Read the model definition and answer for the solid it produces. Units are mm, in the model's axes. Face numbers are marked on the shaded views. Coordinates: 2 decimals unless noted, no trailing zeros. Loops run counter-clockwise (first coordinate to the right, second up) from the corner with the lowest first, then second, coordinate; pieces in that order, holes last. Notation, with made-up numbers: (-35, -15) - (20, -15) arc R13 ccw to (20, 8) - close; hole circle Ø4 at (-1, 27). An arc over 180 degrees is marked (long way). Use one line per item in the form item = value.
from build123d import *

# Parameters (mm, degrees)
F1_DEPTH = 12.7
F2_DEPTH = 75.692
F4_DEPTH = 12.7


with BuildPart() as f1:
    # F0 (on Top) → F1 (new body)
    with BuildSketch(Plane.XY):
        with BuildLine():
            ThreePointArc((0, 8.0484505981), (5.691113996, 5.691113996), (8.0484505981, 0))
            ThreePointArc((8.0484505981, 0), (5.691113996, -5.691113996), (0, -8.0484505981))
            Line((0, -8.0484505981), (0, -19.3179212511))
            ThreePointArc((0, -19.3179212511), (13.6598331151, -13.6598331151), (19.3179212511, 0))
            ThreePointArc((19.3179212511, 0), (13.6598331151, 13.6598331151), (0, 19.3179212511))
            Line((0, 19.3179212511), (0, 8.0484505981))
        make_face()
        with BuildLine():
            ThreePointArc((0, -8.0484505981), (-8.0484505981, 0), (0, 8.0484505981))
            Line((0, 8.0484505981), (0, 19.3179212511))
            ThreePointArc((0, 19.3179212511), (-19.3179212511, 0), (0, -19.3179212511))
            Line((0, -19.3179212511), (0, -8.0484505981))
        make_face()
        with BuildLine():
            Line((61.3472089171, 19.3179212511), (0, 19.3179212511))
            ThreePointArc((0, 19.3179212511), (13.6598331151, 13.6598331151), (19.3179212511, 0))
            ThreePointArc((19.3179212511, 0), (13.6598331151, -13.6598331151), (0, -19.3179212511))
            Line((0, -19.3179212511), (61.3472089171, -19.3179212511))
            ThreePointArc((61.3472089171, -19.3179212511), (42.0292876661, 0), (61.3472089171, 19.3179212511))
        make_face()
        with BuildLine():
            ThreePointArc((80.6651301682, 0), (75.0070420322, 13.6598331151), (61.3472089171, 19.3179212511))
            Line((61.3472089171, 19.3179212511), (61.3472089171, 8.0518))
            ThreePointArc((61.3472089171, 8.0518), (67.0406912979, 5.6934823808), (69.3990089171, 0))
            ThreePointArc((69.3990089171, 0), (67.0406912979, -5.6934823808), (61.3472089171, -8.0518))
            Line((61.3472089171, -8.0518), (61.3472089171, -19.3179212511))
            ThreePointArc((61.3472089171, -19.3179212511), (75.0070420322, -13.6598331151), (80.6651301682, 0))
        make_face()
        with BuildLine():
            Line((61.3472089171, 8.0518), (61.3472089171, 19.3179212511))
            ThreePointArc((61.3472089171, 19.3179212511), (42.0292876661, 0), (61.3472089171, -19.3179212511))
            Line((61.3472089171, -19.3179212511), (61.3472089171, -8.0518))
            ThreePointArc((61.3472089171, -8.0518), (53.2954089171, 0), (61.3472089171, 8.0518))
        make_face()
    extrude(amount=F1_DEPTH)

    # F0 (on Top) → F2 (join)
    with BuildSketch(Plane.XY):
        with BuildLine():
            ThreePointArc((0, -8.0484505981), (-8.0484505981, 0), (0, 8.0484505981))
            Line((0, 8.0484505981), (0, 19.3179212511))
            ThreePointArc((0, 19.3179212511), (-19.3179212511, 0), (0, -19.3179212511))
            Line((0, -19.3179212511), (0, -8.0484505981))
        make_face()
        with BuildLine():
            ThreePointArc((0, 8.0484505981), (5.691113996, 5.691113996), (8.0484505981, 0))
            ThreePointArc((8.0484505981, 0), (5.691113996, -5.691113996), (0, -8.0484505981))
            Line((0, -8.0484505981), (0, -19.3179212511))
            ThreePointArc((0, -19.3179212511), (13.6598331151, -13.6598331151), (19.3179212511, 0))
            ThreePointArc((19.3179212511, 0), (13.6598331151, 13.6598331151), (0, 19.3179212511))
            Line((0, 19.3179212511), (0, 8.0484505981))
        make_face()
    extrude(amount=F2_DEPTH)

    # F3 (on face) → F4 (join)
    with BuildSketch(Plane.XY.offset(75.692)):
        with BuildLine():
            ThreePointArc((19.3179212511, 0), (13.6598331151, 13.6598331151), (0, 19.3179212511))
            Line((0, 19.3179212511), (0, 8.0518))
            ThreePointArc((0, 8.0518), (5.6934823808, 5.6934823808), (8.0518, 0))
            ThreePointArc((8.0518, 0), (5.6934823808, -5.6934823808), (0, -8.0518))
            Line((0, -8.0518), (0, -19.3154787489))
            Line((0, -19.3154787489), (0.3071842465, -19.3154787489))
            ThreePointArc((0.3071842465, -19.3154787489), (13.7680107958, -13.5507918658), (19.3179212511, 0))
        make_face()
        with BuildLine():
            Line((61.341, 19.3179212511), (0, 19.3179212511))
            ThreePointArc((0, 19.3179212511), (13.6598331151, 13.6598331151), (19.3179212511, 0))
            ThreePointArc((19.3179212511, 0), (13.7680107958, -13.5507918658), (0.3071842465, -19.3154787489))
            Line((0.3071842465, -19.3154787489), (61.341, -19.3154787489))
            ThreePointArc((61.341, -19.3154787489), (42.0243, 0.0012212511), (61.341, 19.3179212511))
        make_face()
        with BuildLine():
            Line((0, 8.0518), (0, 19.3179212511))
            ThreePointArc((0, 19.3179212511), (-19.3173106159, -0.1535969784), (0.3071842465, -19.3154787489))
            Line((0.3071842465, -19.3154787489), (0, -19.3154787489))
            Line((0, -19.3154787489), (0, -8.0518))
            ThreePointArc((0, -8.0518), (-8.0518, 0), (0, 8.0518))
        make_face()
        with BuildLine():
            ThreePointArc((80.6577, 0.0012212511), (74.9999695601, 13.6601908112), (61.341, 19.3179212511))
            Line((61.341, 19.3179212511), (61.341, 8.0530212511))
            ThreePointArc((61.341, 8.0530212511), (67.0344823808, 5.6947036318), (69.3928, 0.0012212511))
            ThreePointArc((69.3928, 0.0012212511), (67.0344823808, -5.6922611297), (61.341, -8.0505787489))
            Line((61.341, -8.0505787489), (61.341, -19.3154787489))
            ThreePointArc((61.341, -19.3154787489), (74.9999695601, -13.6577483091), (80.6577, 0.0012212511))
        make_face()
        with BuildLine():
            Line((61.341, 8.0530212511), (61.341, 19.3179212511))
            ThreePointArc((61.341, 19.3179212511), (42.0243, 0.0012212511), (61.341, -19.3154787489))
            Line((61.341, -19.3154787489), (61.341, -8.0505787489))
            ThreePointArc((61.341, -8.0505787489), (53.2892, 0.0012212511), (61.341, 8.0530212511))
        make_face()
    extrude(amount=-F4_DEPTH)


solid = f1.part
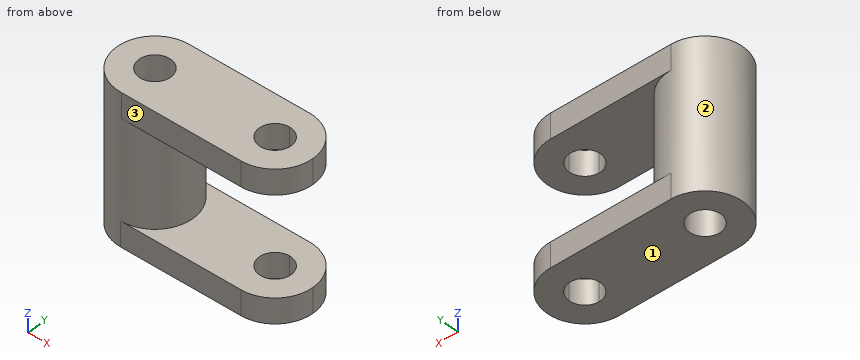
Item 1: The part is cut by section A-A on x = 20.5. Give the vertices of the cut face in (y, z).
Results below:
outline = (-19.32, 0) - (19.32, 0) - (19.32, 12.7) - (-19.32, 12.7) - close; (-19.32, 62.99) - (19.32, 62.99) - (19.32, 75.69) - (-19.32, 75.69) - close
Item 2: For a pull along Z with two mould halves and no side action, classify the marked faces 1, 2 and 3 as +Z half, -Z half, draft (parallel to the pull), parting line (faces both ways), or undercut.
Results below:
face_1 = -Z half
face_2 = undercut
face_3 = draft
Item 3: Find the intervals of material crossed by L1, parallel to X at y = 0, z = 28; L2, parallel to Z at x = 24, y = -16; L3, parallel to X at y = 4, z = 31, in increasing order.
Results below:
L1 = -19.32 to -8.05, 8.05 to 19.32
L2 = 0 to 12.7, 62.99 to 75.69
L3 = -18.9 to -6.98, 6.98 to 18.9
Item 4: The part is cut by section B-B on y = -5. Give the vertices of the cut face in (x, z).
Results below:
outline = (-18.66, 0) - (-6.31, 0) - (-6.31, 75.69) - (-18.66, 75.69) - close; (6.31, 0) - (55.04, 0) - (55.04, 12.7) - (18.66, 12.7) - (18.66, 62.99) - (55.03, 62.99) - (55.03, 75.69) - (6.31, 75.69) - close; (67.65, 62.99) - (80, 62.99) - (80, 75.69) - (67.65, 75.69) - close; (67.66, 0) - (80.01, 0) - (80.01, 12.7) - (67.66, 12.7) - close
Item 5: Each of these flat-tipped pins is pushed along its axis until it touches: P1, Ø1.5, axis at x = -3, z = 38.5, coming from the -Y side; P2, Ø6, axis at y = -11, z = 39, coming from the -X side; P3, Ø14, axis at x = 25.5, z = 71, coming from the -Y side. Where does it stop, or does it pass through?
Results below:
P1 = -19.19
P2 = -17.58
P3 = -19.32
Item 6: The part is cut by section D-D on y = 16. Give the vertices of the cut face in (x, z), plus the area to 3 significant figures.
Results below:
outline = (-10.83, 0) - (72.17, 0) - (72.17, 12.7) - (10.83, 12.7) - (10.83, 62.99) - (72.17, 62.99) - (72.17, 75.69) - (-10.83, 75.69) - close
area = 3,200 mm²
Item 7: The part is cut by section C-C on z = 52. Give the vertices of the cut face in (x, y), plus the area to 3 significant figures.
Results below:
outline = circle Ø38.64 at (0, 0); hole circle Ø16.1 at (0, 0)
area = 969 mm²
